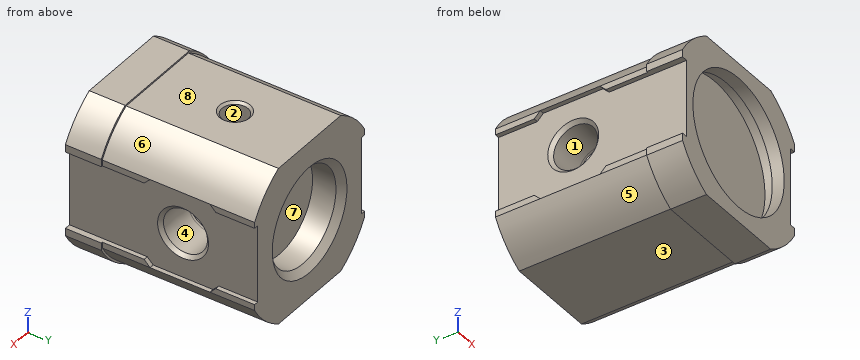
```python
from build123d import *

# Parameters (mm, degrees)
EXTRUDE_1_DEPTH     = 63
EXTRUDE_2_DEPTH     = 12
CUT_EXTRUDE_1_DEPTH = 2
CUT_EXTRUDE_2_DEPTH = 2


with BuildPart() as part:
    # Sketch 1 → Extrude 1 (new body)
    with BuildSketch(Plane(origin=(0, 0, 0), x_dir=(1, 0, 0), z_dir=(0, 1, 0))):
        with BuildLine():
            Line((-26.5, 15), (-26.5, -15))
            ThreePointArc((-26.5, -15), (-21.531953, -21.531953), (-15, -26.5))
            Line((-15, -26.5), (15, -26.5))
            ThreePointArc((15, -26.5), (21.531953, -21.531953), (26.5, -15))
            Line((26.5, -15), (26.5, 15))
            ThreePointArc((26.5, 15), (21.531953, 21.531953), (15, 26.5))
            Line((15, 26.5), (-15, 26.5))
            ThreePointArc((-15, 26.5), (-21.531953, 21.531953), (-26.5, 15))
        make_face()
    extrude(amount=EXTRUDE_1_DEPTH)

    # Sketch 2 → Extrude 2 (add)
    with BuildSketch(Plane(origin=(0, 0, 0), x_dir=(1, 0, 0), z_dir=(0, 1, 0))):
        with BuildLine():
            Line((-27, 15.5), (-27, -15.5))
            ThreePointArc((-27, -15.5), (-22.014199963, -22.014199963), (-15.5, -27))
            Line((-15.5, -27), (15.5, -27))
            ThreePointArc((15.5, -27), (22.014199963, -22.014199963), (27, -15.5))
            Line((27, -15.5), (27, 15.5))
            ThreePointArc((27, 15.5), (22.014199963, 22.014199963), (15.5, 27))
            Line((15.5, 27), (-15.5, 27))
            ThreePointArc((-15.5, 27), (-22.014199963, 22.014199963), (-27, 15.5))
        make_face()
    extrude(amount=EXTRUDE_2_DEPTH)

    # Sketch 3 → Cut-Extrude 1 (cut)
    with BuildSketch(Plane(origin=(-27, 0, 0), x_dir=(0, 0, -1), z_dir=(1, 0, 0))):
        Polygon((-15, 48), (-15, 28), (-13, 26), (-13, 0), (13, 0), (13, 26), (15, 28), (15, 48), (13, 50), (13, 63), (-13, 63), (-13, 50), align=None)
    extrude(amount=CUT_EXTRUDE_1_DEPTH, mode=Mode.SUBTRACT)

    # Sketch 4 → Cut-Extrude 2 (cut)
    with BuildSketch(Plane(origin=(27, 0, 0), x_dir=(0, 0, -1), z_dir=(1, 0, 0))):
        Polygon((-15, 48), (-15, 28), (-13, 26), (-13, 0), (13, 0), (13, 26), (15, 28), (15, 48), (13, 50), (13, 63), (-13, 63), (-13, 50), align=None)
    extrude(amount=-CUT_EXTRUDE_2_DEPTH, mode=Mode.SUBTRACT)

    # Sketch 5 → Cut-Revolve 1 (revolve, cut)
    with BuildSketch(Plane.XY, mode=Mode.PRIVATE) as cut_revolve_1_sk:
        Polygon((0, 63), (18, 63), (15.835, 60.835), (15.835, 53), (0, 53), align=None)
    revolve(cut_revolve_1_sk.sketch.rotate(Axis((0, 53, 0), (0, 1, 0)), 270), axis=Axis((0, 53, 0), (0, 1, 0)), mode=Mode.SUBTRACT)

    # Sketch 6 → Cut-Revolve 2 (revolve, cut)
    with BuildSketch(Plane.XY, mode=Mode.PRIVATE) as cut_revolve_2_sk:
        Polygon((0, 8), (24.25, 8), (24.25, 4), (22, 4), (22, 0), (0, 0), align=None)
    revolve(cut_revolve_2_sk.sketch.rotate(Axis((0, 0, 0), (0, 1, 0)), 270), axis=Axis((0, 0, 0), (0, 1, 0)), mode=Mode.SUBTRACT)

    # Sketch 7 → Cut-Revolve 3 (revolve, cut)
    with BuildSketch(Plane.XY, mode=Mode.PRIVATE) as cut_revolve_3_sk:
        Polygon((-25, 38), (-25, 46.52745952), (-23.834216348, 45.361675868), (-12.573965271, 45.009775437), (-11.783762402, 45.009775437), (-7.736666667, 38), align=None)
    revolve(cut_revolve_3_sk.sketch.rotate(Axis((-7.736666667, 38, 0), (-1, 0, 0)), 270), axis=Axis((-7.736666667, 38, 0), (-1, 0, 0)), mode=Mode.SUBTRACT)

    # Sketch 8 → Cut-Revolve 4 (revolve, cut)
    with BuildSketch(Plane.XY, mode=Mode.PRIVATE) as cut_revolve_4_sk:
        Polygon((7.736666667, 38), (11.783762402, 45.009775437), (12.573965271, 45.009775437), (23.834216348, 45.361675868), (25, 46.52745952), (25, 38), align=None)
    revolve(cut_revolve_4_sk.sketch.rotate(Axis((25, 38, 0), (-1, 0, 0)), 270), axis=Axis((25, 38, 0), (-1, 0, 0)), mode=Mode.SUBTRACT)

    # Sketch 9 → Cut-Revolve 5 (revolve, cut)
    with BuildSketch(Plane(origin=(0, 0, 0), x_dir=(0, 0, -1), z_dir=(1, 0, 0)), mode=Mode.PRIVATE) as cut_revolve_5_sk:
        Polygon((-26.5, 38), (-26.5, 43.121093906), (-25.712414411, 42.333508317), (-18.399867395, 42.104979803), (-16.804611194, 42.104979803), (-14.4346, 38), align=None)
    revolve(cut_revolve_5_sk.sketch.rotate(Axis((0, 38, 14.4346), (0, 0, 1)), 270), axis=Axis((0, 38, 14.4346), (0, 0, 1)), mode=Mode.SUBTRACT)


solid = part.part
```
Geometry: final body of the model. Coordinates: model frame, mm. Face numbers are marked on the shaded views. A direction names the side the tool comes from. Round coordinates to 2 decimals unless told otherwise and drop trailing zeros. Order: outer loops, then holes, each group sorted by start corner. A loop starts at its lowest first (then second) coordinate and runs counter-clockwise, first axis right, second up. Notation, with made-up numbers: (42.25, 78) -> (75.25, 78) arc R16 ccw to (75.25, 93) -> close; hole circle Ø1 at (16.5, 7). An arc over 180 degrees is marked (long way). Use CSV: the item, a comma, the result in double quotes. Start each with the question number.
1) Material intervals for line 1 along Y through (x, z) = (-12, 0); line 2 along X through (y, z) = (3, 0); line 3 along X through (y, z) = (5.25, 0), sorted ascending. Write a range as from..to.
2) Section A-A (y = 5). Return the cut outline in (x, z), and give its area (3 significant figures).
3) Draft query along X for the marked faces 1, 2 and 3. Return one class per face: +X half, -X half, draft (parallel to the pull), parting line (faces both ways), or undercut.
4) Set-up query: the marked faces 4, 5, 6, 7 and 8. Return all of +Z, -Z, +X, -X, +Y, -Y with unobstructed straight access to the full face (end or side cutting, diameter ignored); none if empty.
5) Section C-C (y = 59.5). Return the cut outline in (x, z) (3 decimals).
6) Section B-B (z = -20.5). Return the cut outline in (x, y), and give its area (3 significant figures).
7) First-contact query: pin 1 Ø1.6 at (y, z) = (56.5, -14.5) entering from -X; pin 2 Ø0.6 at (x, y) = (26, 12.5) entering from +Z; pin 3 Ø4 at (y, z) = (35, -20.5) entering from +X. Flat tips, straight axial feed; report the tip coordinate or a pass-through.
Returned:
1,line 1,"y = 8..30.99, 45.01..53"
1,line 2,"x = -25..-22, 22..25"
1,line 3,"x = -25..-24.25, 24.25..25"
2,outline,"(-27, -15.5) arc R31.13 ccw to (-15.5, -27) -> (15.5, -27) arc R31.13 ccw to (27, -15.5) -> (27, -13) -> (25, -13) -> (25, 13) -> (27, 13) -> (27, 15.5) arc R31.13 ccw to (15.5, 27) -> (-15.5, 27) arc R31.13 ccw to (-27, 15.5) -> (-27, 13) -> (-25, 13) -> (-25, -13) -> (-27, -13) -> close; hole circle Ø48.5 at (0, 0)"
2,area,"747 mm²"
3,face 1,"-X half"
3,face 2,"undercut"
3,face 3,"draft"
4,face 4,"+X"
4,face 5,"-Z, -X, +Y"
4,face 6,"+Z, +X, +Y"
4,face 7,"+Y"
4,face 8,"+Z, +X, -X, +Y"
5,outline,"(-26.5, -15) arc R30.451 ccw to (-15, -26.5) -> (15, -26.5) arc R30.451 ccw to (26.5, -15) -> (26.5, -13) -> (25, -13) -> (25, 13) -> (26.5, 13) -> (26.5, 15) arc R30.451 ccw to (15, 26.5) -> (-15, 26.5) arc R30.451 ccw to (-26.5, 15) -> (-26.5, 13) -> (-25, 13) -> (-25, -13) -> (-26.5, -13) -> close; hole circle Ø31.67 at (0, 0)"
6,outline,"(-23.43, 0) -> (-7.98, 0) -> (-7.98, 4) -> (-12.95, 4) -> (-12.95, 8) -> (12.95, 8) -> (12.95, 4) -> (7.98, 4) -> (7.98, 0) -> (23.43, 0) -> (23.43, 12) -> (22.52, 12) -> (22.52, 63) -> (-22.52, 63) -> (-22.52, 12) -> (-23.43, 12) -> close"
6,area,"2,690 mm²"
7,pin 1,"stops at x = -26.5"
7,pin 2,"stops at z = 16.33"
7,pin 3,"stops at x = 24.19"
